For this review, take the finished solid that the model builds, in its own axes (mm). A direction names the side the tool comes from. Coordinates: 2 decimals unless noted, no trailing zeros. Loops run counter-clockwise (first coordinate to the right, second up) from the corner with the lowest first, then second, coordinate; pieces in that order, holes last. Notation, with made-up numbers: (-33, 46) - (-16, 46) arc R22 cw to (-16, 70) - close; hole circle Ø10 at (33, -13.75). An arc over 180 degrees is marked (long way). One line per item, written item: value. Start each with the question number.
1. Insertion check: pin 1 (8 mm diameter, centred on y = 1.5, z = -6.5, fed in from +X); pin 2 (1 mm diameter, centred on y = 13.5, z = -7.5, fed in from -X); pin 3 (6 mm diameter, centred on x = 13, z = -3.5, fed in from +Y). Each pin has a flat end and moves straight along its axis. Give the tip position at first contact, or say it passes through.
2. For faces 1 (the face through (52, 17, -9)), 2 (the face through (44.4, 8, -9)), 3 (the face through (-1.3, 11.45, -6.07)), list the 3-axis set-ups (+Z, -Z, +X, -X, +Y, -Y) from which the entire face can be reached by the end or side of a thin tool; tool diameter is ignored.
3. Take a section at A-A, the plane z = -9.15. State the section outline as (x, y) points, and give its area (3 significant figures).
4. Take a section at B-B, the plane x = 32.2. State the section outline as (y, z) points, and give its area (3 significant figures).
5. Take a section at C-C, the plane y = 9.5. State the section outline as (x, z) points (3 decimals), and give its area (3 significant figures).
6. Take a section at D-D, the plane z = -15.25. State the section outline as (x, y) points.
7. To check wall thickness, follow line 1 (X direction, y = 10.5, z = -16.75); line 2 (X direction, y = 3.75, z = -12.25); line 3 (X direction, y = 14, z = -9). State the ranges of each line that lie inside material, in increasing order. Write a range as from..to.
8. The part is to be moulded in two halves that separate along X. For faces 4 (the face through (-13.289, 15.196, -9.278)), 5 (the face through (57.689, 15.196, -9.278)), 6 (the face through (46.204, 15.289, -9.278)), say which applies: released by +X, released by -X, zero draft, split by the parting line, or undercut.
```python
from build123d import *

# Parameters (mm, degrees)
SKETCH1_W           = 15
SKETCH1_H           = 18.3
SKETCH1_W_2         = 44.4
SKETCH1_R           = 2.15
BOSS_EXTRUDE1_DEPTH = 2
SKETCH1_3_W         = 15
SKETCH1_3_H         = 18.3
BOSS_EXTRUDE2_DEPTH = 17
SKETCH2_R           = 6.5
CUT_EXTRUDE2_DEPTH  = 12.315
FILLET3_R           = 6
FILLET4_R           = 3


with BuildPart() as part:
    # Sketch1 → Boss-Extrude1 (new body)
    # profile 1 of 3: a face of its own
    with BuildSketch(Plane(origin=(0, 0, 0), x_dir=(1, 0, 0), z_dir=(0, 1, 0))):
        with Locations((-7.5, 9.15)):
            Rectangle(SKETCH1_W, SKETCH1_H)
    # profile 2 of 3: a face of its own
    with BuildSketch(Plane(origin=(0, 0, 0), x_dir=(1, 0, 0), z_dir=(0, 1, 0))):
        with Locations((22.2, 9.15)):
            Rectangle(SKETCH1_W_2, SKETCH1_H)
        with Locations(Location((32.2, 9.15, 0), (0, 0, 270))):
            Circle(SKETCH1_R, mode=Mode.SUBTRACT)
        with Locations(Location((12.2, 9.15, 0), (0, 0, 270))):
            Circle(SKETCH1_R, mode=Mode.SUBTRACT)
    # profile 3 of 3: a face of its own
    with BuildSketch(Plane(origin=(0, 0, 0), x_dir=(1, 0, 0), z_dir=(0, 1, 0))):
        with Locations((51.9, 9.15)):
            Rectangle(SKETCH1_W, SKETCH1_H)
    extrude(amount=BOSS_EXTRUDE1_DEPTH)

    # Sketch1<3> → Boss-Extrude2 (add)
    with BuildSketch(Plane(origin=(0, 0, 0), x_dir=(1, 0, 0), z_dir=(0, 1, 0))):
        with Locations((51.9, 9.15)):
            Rectangle(SKETCH1_3_W, SKETCH1_3_H)
        with Locations((-7.5, 9.15)):
            Rectangle(SKETCH1_3_W, SKETCH1_3_H)
    extrude(amount=BOSS_EXTRUDE2_DEPTH)

    # Sketch2 → Cut-Extrude2 (cut)
    with BuildSketch(Plane.XY):
        with Locations((-7.5, 9.5)):
            Circle(SKETCH2_R)
        with Locations((51.9, 9.5)):
            Circle(SKETCH2_R)
    extrude(amount=-CUT_EXTRUDE2_DEPTH, mode=Mode.SUBTRACT)

    # Fillet3
    fillet3_edges = [part.edges().sort_by_distance(p)[0] for p in [
        (59.4, 0, -9.15),
        (-15, 0, -9.15),
        (44.4, 17, -9.15),
        (59.4, 17, -9.15),
        (-15, 17, -9.15),
        (0, 17, -9.15),
    ]]
    fillet(fillet3_edges, radius=FILLET3_R)

    # Fillet4
    fillet4_edges = [part.edges().sort_by_distance(p)[0] for p in [
        (44.4, 2, -9.15),
        (0, 2, -9.15),
    ]]
    fillet(fillet4_edges, radius=FILLET4_R)


solid = part.part
```
Solutions:
1. pin 1: x = 59.38
1. pin 2: x = -14.66
1. pin 3: y = 2
2. face 1: +Z, -Z, +X, -X, +Y
2. face 2: +Z, -Z, +Y
2. face 3: +Z
3. outline: (-15, 6) arc R6 ccw to (-9, 0) - (10.05, 0) - (10.05, 2) - (3, 2) arc R3 cw to (0, 5) - (0, 11) arc R6 ccw to (-6, 17) - (-9, 17) arc R6 ccw to (-15, 11) - close; (14.35, 0) - (30.05, 0) - (30.05, 2) - (14.35, 2) - close; (34.35, 0) - (53.4, 0) arc R6 ccw to (59.4, 6) - (59.4, 11) arc R6 ccw to (53.4, 17) - (50.4, 17) arc R6 ccw to (44.4, 11) - (44.4, 5) arc R3 cw to (41.4, 2) - (34.35, 2) - close; hole circle Ø13 at (-7.5, 9.5); hole circle Ø13 at (51.9, 9.5)
3. area: 274 mm2
4. outline: (0, -18.3) - (2, -18.3) - (2, -11.3) - (0, -11.3) - close; (0, -7) - (2, -7) - (2, 0) - (0, 0) - close
4. area: 28.0 mm2
5. outline: (-15, -18.3) - (0, -18.3) - (0, 0) - (-1, 0) - (-1, -12.315) - (-14, -12.315) - (-14, 0) - (-15, 0) - close; (44.4, -18.3) - (59.4, -18.3) - (59.4, 0) - (58.4, 0) - (58.4, -12.315) - (45.4, -12.315) - (45.4, 0) - (44.4, 0) - close
5. area: 229 mm2
6. outline: (-15, 6) arc R6 ccw to (-9, 0) - (53.4, 0) arc R6 ccw to (59.4, 6) - (59.4, 11) arc R6 ccw to (53.4, 17) - (50.4, 17) arc R6 ccw to (44.4, 11) - (44.4, 5) arc R3 cw to (41.4, 2) - (3, 2) arc R3 cw to (0, 5) - (0, 11) arc R6 ccw to (-6, 17) - (-9, 17) arc R6 ccw to (-15, 11) - close
7. line 1: -15..0, 44.4..59.4
7. line 2: -14.56..-10.53, -4.47..0.27, 44.13..48.87, 54.93..58.96
7. line 3: -14.2..-12.19, -2.81..-0.8, 45.2..47.21, 56.59..58.6
8. face 4: released by -X
8. face 5: released by +X
8. face 6: undercut
